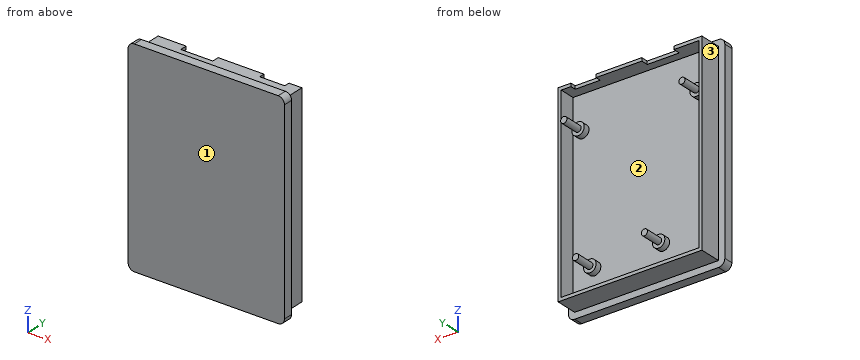
```python
from build123d import *

# Parameters (mm, degrees)
SKETCH1_W           = 63.5
SKETCH1_H           = 83.82
BOSS_EXTRUDE1_DEPTH = 12.7
SKETCH2_W           = 55.88
SKETCH2_H           = 76.2
CUT_EXTRUDE1_DEPTH  = 6.35
SKETCH3_W           = 63.5
SKETCH3_H           = 83.82
SKETCH3_W_2         = 58.42
SKETCH3_H_2         = 78.74
CUT_EXTRUDE2_DEPTH  = 8.89
SKETCH6_R           = 1.27
BOSS_EXTRUDE3_DEPTH = 10.16
SKETCH8_R           = 2.54
BOSS_EXTRUDE4_DEPTH = 2.54
SKETCH10_W          = 13.010391052
SKETCH10_H          = 3.325331773
CUT_EXTRUDE4_DEPTH  = 10.16
SKETCH11_W          = 10.16
SKETCH11_H          = 2.62905351
CUT_EXTRUDE5_DEPTH  = 10.16
FILLET1_R           = 2.54


with BuildPart() as part:
    # Sketch1 → Boss-Extrude1 (new body)
    with BuildSketch(Plane(origin=(0, 0, 0), x_dir=(1, 0, 0), z_dir=(0, 1, 0))):
        Rectangle(SKETCH1_W, SKETCH1_H)
    extrude(amount=BOSS_EXTRUDE1_DEPTH)

    # Sketch2 → Cut-Extrude1 (cut)
    with BuildSketch(Plane(origin=(0, 12.7, 0), x_dir=(1, 0, 0), z_dir=(0, 1, 0))):
        Rectangle(SKETCH2_W, SKETCH2_H)
    extrude(amount=-CUT_EXTRUDE1_DEPTH, mode=Mode.SUBTRACT)

    # Sketch3 → Cut-Extrude2 (cut)
    with BuildSketch(Plane(origin=(0, 12.7, 0), x_dir=(1, 0, 0), z_dir=(0, 1, 0))):
        Rectangle(SKETCH3_W, SKETCH3_H)
        Rectangle(SKETCH3_W_2, SKETCH3_H_2, mode=Mode.SUBTRACT)
    extrude(amount=-CUT_EXTRUDE2_DEPTH, mode=Mode.SUBTRACT)

    # Sketch6 → Boss-Extrude3 (add)
    with BuildSketch(Plane(origin=(0, 6.35, 0), x_dir=(1, 0, 0), z_dir=(0, 1, 0))):
        with Locations(Location((-23.958920987, -23.008465221, 0), (0, 0, 270))):
            Circle(SKETCH6_R)
        with Locations(Location((-8.718920987, 27.778834779, 0), (0, 0, 270))):
            Circle(SKETCH6_R)
        with Locations(Location((19.208379013, 27.778834779, 0), (0, 0, 270))):
            Circle(SKETCH6_R)
        with Locations(Location((24.012870789, -24.225811214, 0), (0, 0, 270))):
            Circle(SKETCH6_R)
    extrude(amount=BOSS_EXTRUDE3_DEPTH)

    # Sketch8 → Boss-Extrude4 (add)
    with BuildSketch(Plane(origin=(0, 6.35, 0), x_dir=(1, 0, 0), z_dir=(0, 1, 0))):
        with Locations(Location((19.208379013, 27.778834779, 0), (0, 0, 270))):
            Circle(SKETCH8_R)
        with Locations(Location((-8.718920987, 27.778834779, 0), (0, 0, 270))):
            Circle(SKETCH8_R)
        with Locations(Location((-23.958920987, -23.008465221, 0), (0, 0, 270))):
            Circle(SKETCH8_R)
        with Locations(Location((24.012870789, -24.225811214, 0), (0, 0, 270))):
            Circle(SKETCH8_R)
    extrude(amount=BOSS_EXTRUDE4_DEPTH)

    # Sketch10 → Cut-Extrude4 (cut)
    with BuildSketch(Plane.XY.offset(39.37)):
        with Locations((-11.303612935, 11.47098091)):
            Rectangle(SKETCH10_W, SKETCH10_H)
    extrude(amount=-CUT_EXTRUDE4_DEPTH, mode=Mode.SUBTRACT)

    # Sketch11 → Cut-Extrude5 (cut)
    with BuildSketch(Plane.XY.offset(39.37)):
        with Locations((18.901215122, 11.759143512)):
            Rectangle(SKETCH11_W, SKETCH11_H)
    extrude(amount=-CUT_EXTRUDE5_DEPTH, mode=Mode.SUBTRACT)

    # Fillet1
    fillet1_edges = [part.edges().sort_by_distance(p)[0] for p in [
        (31.75, 1.905, 41.91),
        (-31.75, 1.905, 41.91),
        (-31.75, 1.905, -41.91),
        (31.75, 1.905, -41.91),
    ]]
    fillet(fillet1_edges, radius=FILLET1_R)


solid = part.part
```
For this review, take the finished solid that the model builds, in its own axes (mm). Face numbers are marked on the shaded views. Coordinates: 2 decimals unless noted, no trailing zeros. Order: outer loops, then holes, each group sorted by start corner. A loop starts at its lowest first (then second) coordinate and runs counter-clockwise, first axis right, second up. Notation, with made-up numbers: (47, 9) -> (79, 9) arc R26 cw to (79, 38) -> close; hole circle Ø2 at (-16, 42.5). An arc over 180 degrees is marked (long way). Use CSV: the item, a comma, the result in double quotes. Start each with the question number.
Item 1: Insertion check: pin 1 (1.5 mm diameter, centred on x = -20, z = -33.5, fed in from -Y); pin 2 (17 mm diameter, centred on x = -0.5, z = -5, fed in from +Y); pin 3 (2.5 mm diameter, centred on y = 7.5, z = 17, fed in from -X); pin 4 (3 mm diameter, centred on x = -7.5, y = 12, fed in from -Z). Each pin has a flat end and moves straight along its axis. Give the tip position at first contact, or say it passes through.
Item 2: We need section B-B, the plane y = 14.5. Give the boundary of the cut face in (x, z), then the cut area to 3 significant figures.
Item 3: We need section A-A, the plane z = 30. Give the boundary of the cut face in (x, y).
Item 4: Draft analysis for pull direction X (two halves, no side actions). For the marked faces 1, 2 and 3, state which applies: pulls with the +X half, pulls with the -X half, needs draft (parallel to the pull), parting line crosses it, or undercut.
Item 5: Wall thickness on probe 1 along X at (y, z) = (10.25, -23.5); probe 2 along Z at (x, y) = (26.5, 10); probe 3 along Y at (x, z) = (-22, -1): over which ranges is each line inside the solid? List them lowest first.
Derived:
1,pin 1,"stops at y = 0"
1,pin 2,"stops at y = 6.35"
1,pin 3,"stops at x = -29.21"
1,pin 4,"stops at z = -39.37"
2,outline,"circle Ø2.54 at (-23.96, 23.01); circle Ø2.54 at (-8.72, -27.78); circle Ø2.54 at (19.21, -27.78); circle Ø2.54 at (24.01, 24.23)"
2,area,"20.3 mm^2"
3,outline,"(-31.75, 0) -> (31.75, 0) -> (31.75, 3.81) -> (29.21, 3.81) -> (29.21, 12.7) -> (27.94, 12.7) -> (27.94, 6.35) -> (-27.94, 6.35) -> (-27.94, 12.7) -> (-29.21, 12.7) -> (-29.21, 3.81) -> (-31.75, 3.81) -> close"
4,face 1,"needs draft"
4,face 2,"undercut"
4,face 3,"pulls with the -X half"
5,probe 1,"x = -29.21 to -27.94, 27.94 to 29.21"
5,probe 2,"z = -39.37 to -38.1, 38.1 to 39.37"
5,probe 3,"y = 0 to 6.35"
